Autodesk Inventor part; units mm, degrees
ref_plane "YZ Plane" through (0, 0, 0) normal (1, 0, 0) x (0, 1, 0)
ref_plane "XZ Plane" through (0, 0, 0) normal (0, 1, 0) x (-1, 0, 0)
ref_plane "XY Plane" through (0, 0, 0) normal (0, 0, 1) x (1, 0, 0)
sketch "Sketch1" plane through (0, 0, 0) normal (0, 1, 0) x (-1, 0, 0)
  line L0 (-60, -84) -> (60, -84)
  line L1 (60, -84) -> (60, 84)
  line L2 (60, 84) -> (-60, 84)
  line L3 (-60, 84) -> (-60, -84)
  line L4 (-60, -84) -> (60, 84) construction
  line L5 (60, -84) -> (-60, 84) construction
  point P0 (0, 0)
  dimension "d0" = 168
  dimension "d1" = 120
extrude "Extrusion1" add sketch "Sketch1" along normal blind 2.4
sketch "Sketch2" plane through (0, 2.4, 0) normal (0, 1, 0) x (1, 0, 0)
  line L0 (60, -84) -> (60, 84)
  line L1 (60, -68.75) -> (57.6, -68.75)
  line L2 (57.6, -68.75) -> (57.6, -51.25)
  line L3 (57.6, -51.25) -> (60, -51.25)
  line L4 (60, -51.25) -> (60, -68.75)
  line L5 (-60, -84) -> (60, -84)
  point P0 (0, 0)
  dimension "d4" = 2.4
  dimension "d5" = 17.5
  dimension "d6" = 15.25
extrude "Extrusion2" add sketch "Sketch2" along normal blind 8.25
sketch "Sketch3" plane through (0, 2.4, 0) normal (0, 1, 0) x (1, 0, 0)
  line L0 (59.425, -52.5) -> (58.175, -52.5)
  line L1 (58.175, -52.5) -> (58.175, -50)
  line L2 (58.175, -50) -> (59.425, -50)
  line L3 (59.425, -50) -> (59.425, -52.5)
  line L4 (57.6, -51.25) -> (60, -51.25)
  line L5 (59.425, -52.5) -> (58.175, -50) construction
  line L6 (58.175, -52.5) -> (59.425, -50) construction
  line L7 (59.425, -67.5) -> (58.175, -67.5)
  line L8 (58.175, -67.5) -> (58.175, -70)
  line L9 (58.175, -70) -> (59.425, -70)
  line L10 (59.425, -70) -> (59.425, -67.5)
  line L11 (60, -68.75) -> (57.6, -68.75)
  line L12 (59.425, -67.5) -> (58.175, -70) construction
  line L13 (58.175, -67.5) -> (59.425, -70) construction
  point P0 (0, 0)
  point P1 (58.8, -51.25)
  point P2 (58.8, -68.75)
  point P3 (59.425, -68.75)
  point P4 (58.175, -68.75)
  point P5 (58.175, -51.25)
  point P6 (59.425, -51.25)
  dimension "d9" = 1.25
  dimension "d10" = 2.5
  dimension "d11" = 1.25
  dimension "d12" = 2.5
extrude "Extrusion3" add sketch "Sketch3" along normal blind 8.25 contours L4 L1 L2 L3 | L10 L9 L8 L11
sketch "Sketch4" plane through (0, 2.4, 0) normal (0, 1, 0) x (1, 0, 0)
  line L0 (60, -84) -> (60, -68.75)
  line L1 (-60, -84) -> (60, -84)
  line L2 (41.5, -71) -> (36.5, -71)
  line L3 (36.5, -71) -> (36.5, -49)
  line L4 (36.5, -49) -> (41.5, -49)
  line L5 (41.5, -49) -> (41.5, -71)
  line L6 (40.3125, -67) -> (37.6875, -67)
  line L7 (37.6875, -67) -> (37.6875, -75)
  line L8 (37.6875, -75) -> (40.3125, -75)
  line L9 (40.3125, -75) -> (40.3125, -67)
  line L10 (40.3125, -67) -> (37.6875, -75) construction
  line L11 (37.6875, -67) -> (40.3125, -75) construction
  line L12 (40.3125, -53) -> (37.6875, -53)
  line L13 (37.6875, -53) -> (37.6875, -45)
  line L14 (37.6875, -45) -> (40.3125, -45)
  line L15 (40.3125, -45) -> (40.3125, -53)
  line L16 (40.3125, -53) -> (37.6875, -45) construction
  line L17 (37.6875, -53) -> (40.3125, -45) construction
  point P0 (0, 0)
  point P1 (39, -71)
  point P2 (39, -49)
  point P3 (40.3125, -71)
  point P4 (37.6875, -71)
  point P5 (37.6875, -49)
  point P6 (40.3125, -49)
  dimension "d15" = 18.5
  dimension "d16" = 13
  dimension "d17" = 5
  dimension "d18" = 22
  dimension "d21" = 2.625
  dimension "d22" = 8
  dimension "d23" = 2.625
  dimension "d24" = 8
extrude "Extrusion4" add sketch "Sketch4" along normal blind 11.25
ref_plane "Work Plane3" through (-60, 0, 0) normal (0, 0, 1) x (1, 0, 0)
sketch "Sketch11" plane through (0, 0, 0) normal (0, -1, 0) x (1, 0, 0)
  line L0 (-60, 84) -> (60, 84)
  line L1 (-60, -84) -> (-60, 84)
  line L2 (60, -84) -> (-60, -84)
  point P0 (0, 0)
  point P1 (-56, 78)
  point P2 (-56, -78)
  dimension "d63" = 6
  dimension "d64" = 4
  dimension "d65" = 4
  dimension "d66" = 6
hole "Hole1" at (-56, 0, 78) at (-56, 0, -78) direction (0, 1, 0) diameter 4 end through all
sketch "Sketch12" plane through (0, 2.4, 0) normal (0, 1, 0) x (1, 0, 0)
  point P0 (0, 0)
sketch "Sketch13" plane through (0, 0, 0) normal (0, -1, 0) x (1, 0, 0)
  line L0 (60, 84) -> (60, -84)
  line L1 (-60, 84) -> (60, 84)
  point P0 (0, 0)
  point P1 (54, 78)
  point P2 (54.2858, -79.2517)
  dimension "d74" = 6
  dimension "d75" = 6
hole "Hole2" at (54, 0, 78) direction (0, 1, 0) diameter 4 depth 10 tip angle 118
mirror "Mirror4" about plane through (-60, 0, 0) normal (0, 0, 1) of "Hole2"
properties part number "lower casing"
Design review of the part built by this model. Coordinates are the model's own, in mm. A direction names the side the tool comes from. Give positions to 0.01 mm unless a question says otherwise; leave off trailing zeros. Write each loop counter-clockwise with the first axis right and the second up, starting at its lowest first coordinate (ties: lowest second). Pieces come first, ordered by that corner, then holes. Notation, with made-up numbers: M -2,31.5 L 33,31.5 A17 cw 33,46.5 Z; hole C 47,12.5 d7. An arc over 180 degrees is marked long. Return JSON: item names as keys, results as strings. Group by question number.
Item 1: Wall thickness on line 1 along X through (y, z) = (1.9, 78); line 2 along Z through (x, y) = (54, 0.95); line 3 along Y through (x, z) = (43.5, -69): over which ranges is each line inside the solid? List them lowest first.
Item 2: Take a section at C-C (x = 54). Give the boundary of the cut face in (y, z).
Item 3: Tool access review of faces 1 (the flat face through (40.312, 8, 73)), 2 (the flat face through (37.688, 8, 73)), 3 (the flat face through (40.312, 8, 47)), 4 (the flat face through (57.6, 6, 60)), 5 (the flat face through (37.688, 8, 47)): name each direction out of +Z, -Z, +X, -X, +Y, -Y from which nothing blocks a thin tool from reaching the whole face with its end or side.
Item 4: Take a section at A-A (z = 78). Give the boundary of the cut face in (x, y), plus the area to 3 significant figures.
Item 5: Take a section at D-D (z = -69.5). Give the boundary of the cut face in (x, y), plus the area to 3 significant figures.
Item 6: Clearance check with flat-ended pins moving along their axes: pin 1 Ø4 at (x, z) = (-24, -64.5) entering from -Y; pin 2 Ø2 at (y, z) = (10, 72.5) entering from +X; pin 3 Ø1.9 at (x, z) = (59, 63) entering from +Y; pin 4 Ø6.5 at (x, z) = (-56, 78) entering from +Y. State where each tip first meets the part, or that it passes through.
Return value:
{
 "1": {"line 1": "x = -60 to -58, -54 to 52, 56 to 60", "line 2": "z = -84 to -80, -76 to 76, 80 to 84", "line 3": "y = 0 to 2.4"},
 "2": {"outline": "M 0,-84 L 2.4,-84 L 2.4,-80 L 0,-80 Z; M 0,-76 L 2.4,-76 L 2.4,76 L 0,76 Z; M 0,80 L 2.4,80 L 2.4,84 L 0,84 Z"},
 "3": {"face 1": "+Z, +X, +Y", "face 2": "+Z, -X, +Y", "face 3": "-Z, +X, +Y", "face 4": "+Z, -Z, +Y", "face 5": "-Z, -X, +Y"},
 "4": {"outline": "M -60,0 L -58,0 L -58,2.4 L -60,2.4 Z; M -54,0 L 52,0 L 52,2.4 L -54,2.4 Z; M 56,0 L 60,0 L 60,2.4 L 56,2.4 Z", "area": "269 mm2"},
 "5": {"outline": "M -60,0 L 60,0 L 60,2.4 L -60,2.4 Z", "area": "288 mm2"},
 "6": {"pin 1": "stops at y = 0", "pin 2": "stops at x = 40.31", "pin 3": "stops at y = 10.65", "pin 4": "stops at y = 2.4"}
}
